Check sheet for the drawn part. Datum: minimum x, y, z corner. Units: mm. A direction names the side the tool comes from. Coordinates: 2 decimals unless noted, no trailing zeros. Loops run counter-clockwise (first coordinate to the right, second up) from the corner with the lowest first, then second, coordinate; pieces in that order, holes last.
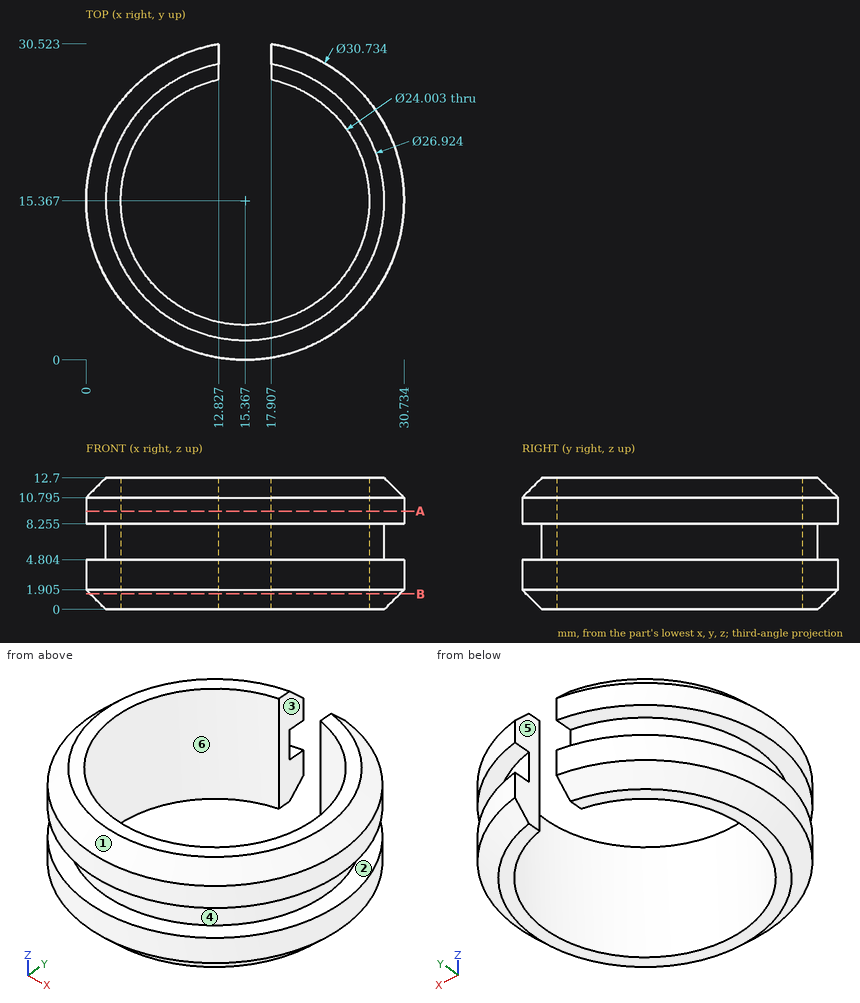
1) Scan lines: line 1 (X direction, y = 16, z = 7); line 2 (X direction, y = 23.5, z = 2.75) (1 decimal); line 3 (Z direction, x = 11.5, y = 2) (1 decimal). Record each from-to range of solid material in increasing order.
Answer sheet:
line 1: x = 1.92 to 3.38, 27.35 to 28.81
line 2: x = 2.3 to 6.5, 24.2 to 28.4
line 3: z = 0.5 to 4.8, 8.3 to 12.2
2) Mould release check, pull along Z, two halves, no side actions. Record for the marked faces 1, 2 and 3: +Z half, -Z half, draft (parallel to the pull), parting line (faces both ways), or undercut.
Answer sheet:
face 1: +Z half
face 2: undercut
face 3: draft
3) Depth check by flat-ended pin: pin 1 (1.5 mm diameter, centred on x = 25.5, y = 22, fed in from -Z); pin 2 (1 mm diameter, centred on x = 23.5, z = 5.5, fed in from +Y) (1 decimal); pin 3 (2 mm diameter, centred on x = 23.5, z = 3, fed in from +Y); pin 4 (4 mm diameter, centred on y = 29, z = 4, fed in from +X). Enter the tip coordinate at first touch or a pass-through.
Answer sheet:
pin 1: stops at z = 0
pin 2: stops at y = 26.5
pin 3: stops at y = 28.98
pin 4: stops at x = 25.41
4) Section check B-B on z = 1.5. Enter the section's corners in (x, y).
Answer sheet:
outline: (12.83, 27.1) - (12.83, 30.11) arc R14.96 ccw (long way) to (17.91, 30.11) - (17.91, 27.1) arc R12 cw (long way) to start
5) Section check A-A on z = 9.5. Enter the section's corners in (x, y), plus the area to 3 significant figures.
Answer sheet:
outline: (12.83, 27.1) - (12.83, 30.52) arc R15.37 ccw (long way) to (17.91, 30.52) - (17.91, 27.1) arc R12 cw (long way) to start
area: 272 mm2
6) Set-up check for the marked faces 4, 5 and 6: record each of +Z, -Z, +X, -X, +Y, -Y from which the full face is reachable in a straight line by a thin tool's end or side.
Answer sheet:
face 4: none
face 5: +Z, -Z, +Y
face 6: +Z, -Z
